Part print with two shaded views. Sizes in mm from the minimum x, y, z corner. Round coordinates to 2 decimals unless told otherwise and drop trailing zeros. Write each loop counter-clockwise with the first axis right and the second up, starting at its lowest first coordinate (ties: lowest second). Pieces come first, ordered by that corner, then holes. Notation, with made-up numbers: (73, 62.5) -> (85, 62.5) arc R8 cw to (85, 71.5) -> close; hole circle Ø5 at (-17, 11.5). An arc over 180 degrees is marked (long way). Return JSON: item names as keys, results as strings.
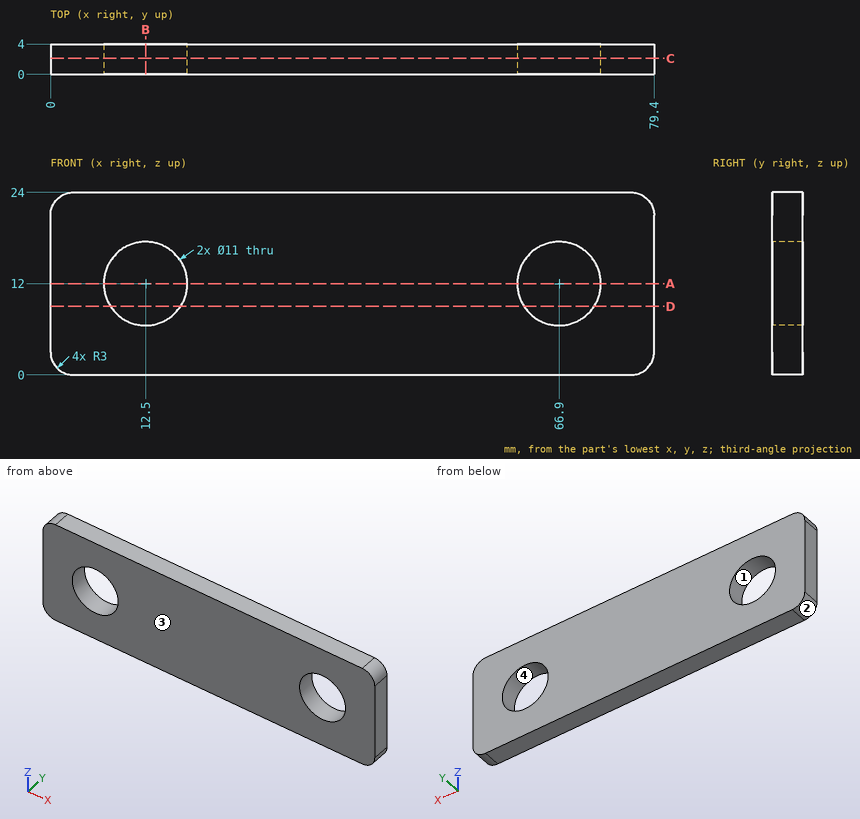
Q1. Saw through at B-B on x = 12.5. List the corners of the cut face in (y, z), then the cut area to 3 significant figures.
Verdict:
{"outline": "(0, 0) -> (4, 0) -> (4, 6.5) -> (0, 6.5) -> close; (0, 17.5) -> (4, 17.5) -> (4, 24) -> (0, 24) -> close", "area": "52.0 mm²"}
Q2. Two-plate mould, pull along Z, no slides. Class the marked faces 1, 2, 3 and 4: +Z half, -Z half, draft (parallel to the pull), parting line (faces both ways), or undercut.
Verdict:
{"face 1": "undercut", "face 2": "-Z half", "face 3": "draft", "face 4": "undercut"}
Q3. Saw through at A-A on z = 12. List the corners of the cut face in (x, y), then the cut area to 3 significant figures.
Verdict:
{"outline": "(0, 0) -> (7, 0) -> (7, 4) -> (0, 4) -> close; (18, 0) -> (61.4, 0) -> (61.4, 4) -> (18, 4) -> close; (72.4, 0) -> (79.4, 0) -> (79.4, 4) -> (72.4, 4) -> close", "area": "230 mm²"}
Q4. Wall check: L1, parallel to X at y = 0.25, z = 15.25; L2, parallel to Z at x = 66.9, y = 3.2; L3, parallel to X at y = 0.9, z = 9.75. Give the ranges that are in metal, low to high.
Verdict:
{"L1": "x = 0 to 8.06, 16.94 to 62.46, 71.34 to 79.4", "L2": "z = 0 to 6.5, 17.5 to 24", "L3": "x = 0 to 7.48, 17.52 to 61.88, 71.92 to 79.4"}
Q5. Saw through at D-D on z = 9. List the corners of the cut face in (x, y), then the cut area to 3 significant figures.
Verdict:
{"outline": "(0, 0) -> (7.89, 0) -> (7.89, 4) -> (0, 4) -> close; (17.11, 0) -> (62.29, 0) -> (62.29, 4) -> (17.11, 4) -> close; (71.51, 0) -> (79.4, 0) -> (79.4, 4) -> (71.51, 4) -> close", "area": "244 mm²"}
Q6. Pin check, flat tips, straight feed: pin 1 Ø9 at (x, z) = (66.9, 12) entering from -Y; pin 2 Ø6 at (x, z) = (59.5, 9.5) entering from -Y. Stop position of each tip, or through.
Verdict:
{"pin 1": "passes through", "pin 2": "stops at y = 0"}
Q7. Saw through at C-C on y = 2.1. List the corners of the cut face in (x, z).
Verdict:
{"outline": "(0, 3) arc R3 ccw to (3, 0) -> (76.4, 0) arc R3 ccw to (79.4, 3) -> (79.4, 21) arc R3 ccw to (76.4, 24) -> (3, 24) arc R3 ccw to (0, 21) -> close; hole circle Ø11 at (12.5, 12); hole circle Ø11 at (66.9, 12)"}
